Job drawing, mm, ordinate dimensions from the low corner. One solid piece. A direction names the side the tool comes from. Round coordinates to 2 decimals unless told otherwise and drop trailing zeros. Write each loop counter-clockwise with the first axis right and the second up, starting at its lowest first coordinate (ties: lowest second). Pieces come first, ordered by that corner, then holes.
1) Saw through at D-D on y = 94. Write the cut outline in (x, z).
2) Drill centre lines: L1, parallel to Y at x = 27, z = 5; L2, parallel to X at y = 68, z = 2.75; L3, parallel to Y at x = 37.5, z = 6. Where is each one in solid material? Low to high.
3) Saw through at B-B on x = 39. Write the cut outline in (y, z) (1 decimal).
4) Saw through at C-C on z = 4.5. Write the cut outline in (x, y).
5) Saw through at A-A on x = 27. Write the cut outline in (y, z), and give its area (3 significant figures).
6) Which spindle directions (+Z, -Z, +X, -X, +Y, -Y) get a long thin tool onto all of the face, cutting with end or side? Do the marked faces 1, 2 and 3. Say none if no direction does.
7) Flat gauge pins, fed straight in: pin 1 (4 mm diameter, centred on x = 45.5, z = 5.5, fed in from +Y); pin 2 (6 mm diameter, centred on x = 46.5, y = 97.5, fed in from +Z); pin 3 (3 mm diameter, centred on x = 38.5, z = 7.5, fed in from +Y). Where does each tip first touch, or does it go through?
8) Pull direction X, two halves, no side cores. Call the marked faces 4, 5 and 6: +X half, -X half, draft (parallel to the pull), parting line (faces both ways), or undercut.
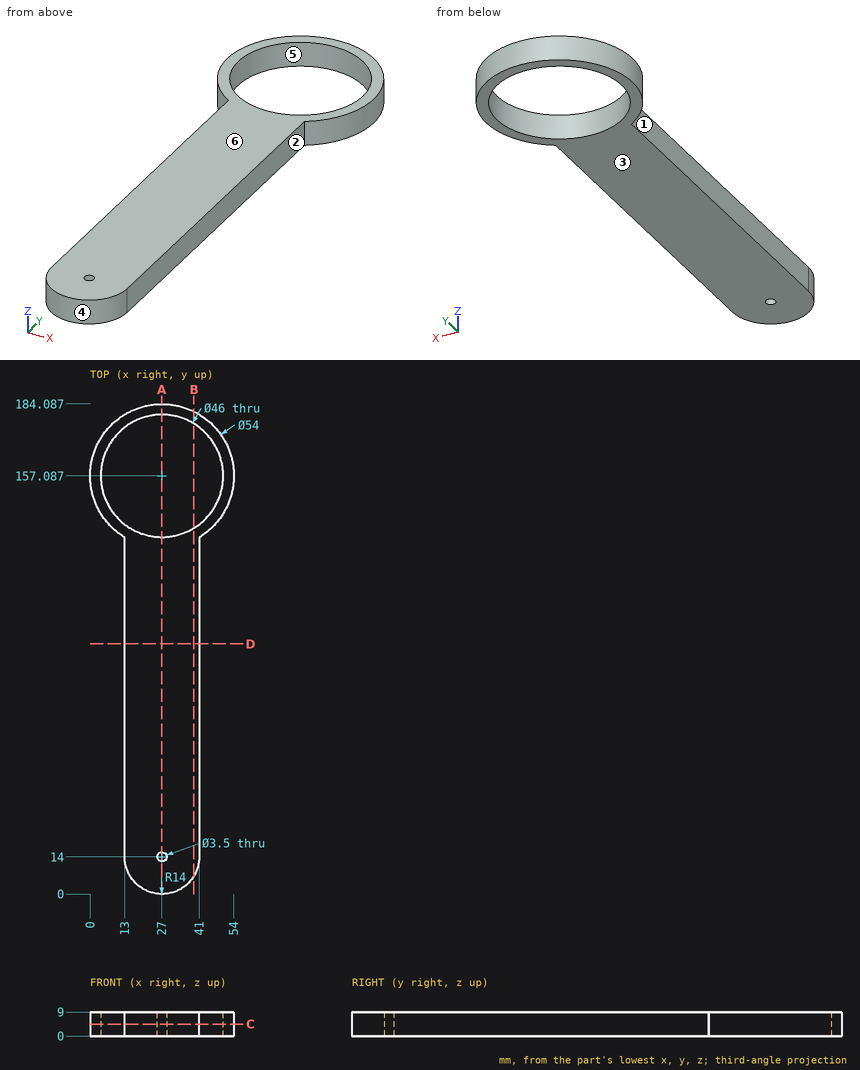
Completed:
1. outline: (13, 0) - (41, 0) - (41, 9) - (13, 9) - close
2. L1: y = 0 to 12.25, 15.75 to 134.09, 180.09 to 184.09
2. L2: x = 13 to 41
2. L3: y = 4.74 to 136.62, 177.55 to 181.96
3. outline: (6.8, 0) - (137.5, 0) - (137.5, 9) - (6.8, 9) - close; (176.7, 0) - (181.3, 0) - (181.3, 9) - (176.7, 9) - close
4. outline: (13, 14) arc R14 ccw to (41, 14) - (41, 134) arc R27 ccw (long way) to (13, 134) - close; hole circle Ø46 at (27, 157.09); hole circle Ø3.5 at (27, 14)
5. outline: (0, 0) - (12.25, 0) - (12.25, 9) - (0, 9) - close; (15.75, 0) - (134.09, 0) - (134.09, 9) - (15.75, 9) - close; (180.09, 0) - (184.09, 0) - (184.09, 9) - (180.09, 9) - close
5. area: 1,210 mm2
6. face 1: +Z, -Z, -X, -Y
6. face 2: +Z, -Z, +X, -Y
6. face 3: -Z, +X, -X, +Y, -Y
7. pin 1: stops at y = 178.46
7. pin 2: passes through
7. pin 3: stops at y = 182.17
8. face 4: parting line
8. face 5: undercut
8. face 6: draft
